Answer from the drawing. Dimensions are ordinates in mm from the lowest x, y and z of the part. A direction names the side the tool comes from. Give positions to 0.01 mm unless a question says otherwise; leave off trailing zeros. Loops run counter-clockwise (first coordinate to the right, second up) from the corner with the lowest first, then second, coordinate; pieces in that order, holes last.
Item 1: Each of these flat-tipped pins is pushed along its axis until it touches: pin 1 Ø5.5 at (x, z) = (4, 10.74) entering from -Y; pin 2 Ø12 at (x, y) = (33.5, 20.5) entering from +Z; pin 3 Ø1.2 at (y, z) = (20.5, 1.5) entering from -X. Where does it stop, or does it pass through?
Item 2: The mould has two halves that part along X. Classify the marked faces 4, 5 and 6: pulls with the +X half, pulls with the -X half, needs draft (parallel to the pull), parting line crosses it, or undercut.
Item 3: Section B-B, the plane x = 40.5 is taken. Give the vertices of the cut face in (y, z).
Item 4: Section A-A, the plane y = 13 is taken. Give the vertices of the cut face in (x, z) (1 decimal).
Item 5: A tool of negligible diameter and unlimited length cuts with its end or side. For the marked faces 1, 2 and 3, from which of +Z, -Z, +X, -X, +Y, -Y can it reach the whole face along a straight path? Write none if from no direction.
Item 6: Consider line 1 along X through (y, z) = (27.5, 3.25) (1 decimal); line 2 along Y through (x, z) = (2, 8.5); line 3 along Y through (x, z) = (41.5, 3.9) (1 decimal). Determine where each line is inside the solid, lowest interval first.
Item 7: Section D-D, the plane x = 22.5 is taken. Give the vertices of the cut face in (y, z) (1 decimal).
Item 8: Section C-C, the plane y = 19 is taken. Give the vertices of the cut face in (x, z) (1 decimal).
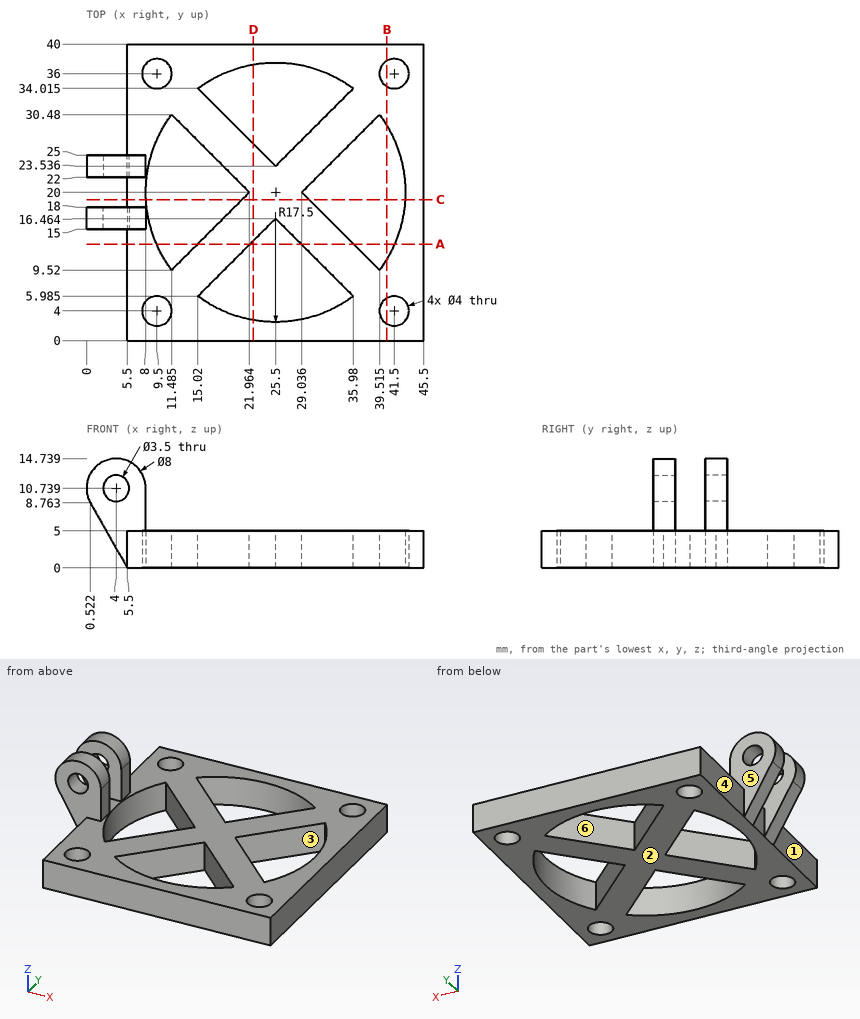
Worked answers:
1. pin 1: stops at y = 15
1. pin 2: stops at z = 5
1. pin 3: stops at x = 5.5
2. face 4: pulls with the -X half
2. face 5: needs draft
2. face 6: undercut
3. outline: (0, 0) - (2.27, 0) - (2.27, 5) - (0, 5) - close; (5.73, 0) - (10.99, 0) - (10.99, 5) - (5.73, 5) - close; (29.01, 0) - (34.27, 0) - (34.27, 5) - (29.01, 5) - close; (37.73, 0) - (40, 0) - (40, 5) - (37.73, 5) - close
4. outline: (5.5, 0) - (9.5, 0) - (9.5, 5) - (5.5, 5) - close; (15, 0) - (22, 0) - (22, 5) - (15, 5) - close; (29, 0) - (36, 0) - (36, 5) - (29, 5) - close; (41.5, 0) - (45.5, 0) - (45.5, 5) - (41.5, 5) - close
5. face 1: +Z, -Z, -X, -Y
5. face 2: -Z, +X, -X, +Y, -Y
5. face 3: +Z, -Z
6. line 1: x = 5.5 to 9.7, 14.5 to 21.5, 29.5 to 36.5, 41.3 to 45.5
6. line 2: y = 15 to 18, 22 to 25
6. line 3: y = 0 to 2, 6 to 12.9, 27.1 to 34, 38 to 40
7. outline: (0, 0) - (2.8, 0) - (2.8, 5) - (0, 5) - close; (13.5, 0) - (26.5, 0) - (26.5, 5) - (13.5, 5) - close; (37.2, 0) - (40, 0) - (40, 5) - (37.2, 5) - close
8. outline: (5.5, 0) - (8, 0) - (8, 5) - (5.5, 5) - close; (21, 0) - (30, 0) - (30, 5) - (21, 5) - close; (43, 0) - (45.5, 0) - (45.5, 5) - (43, 5) - close
